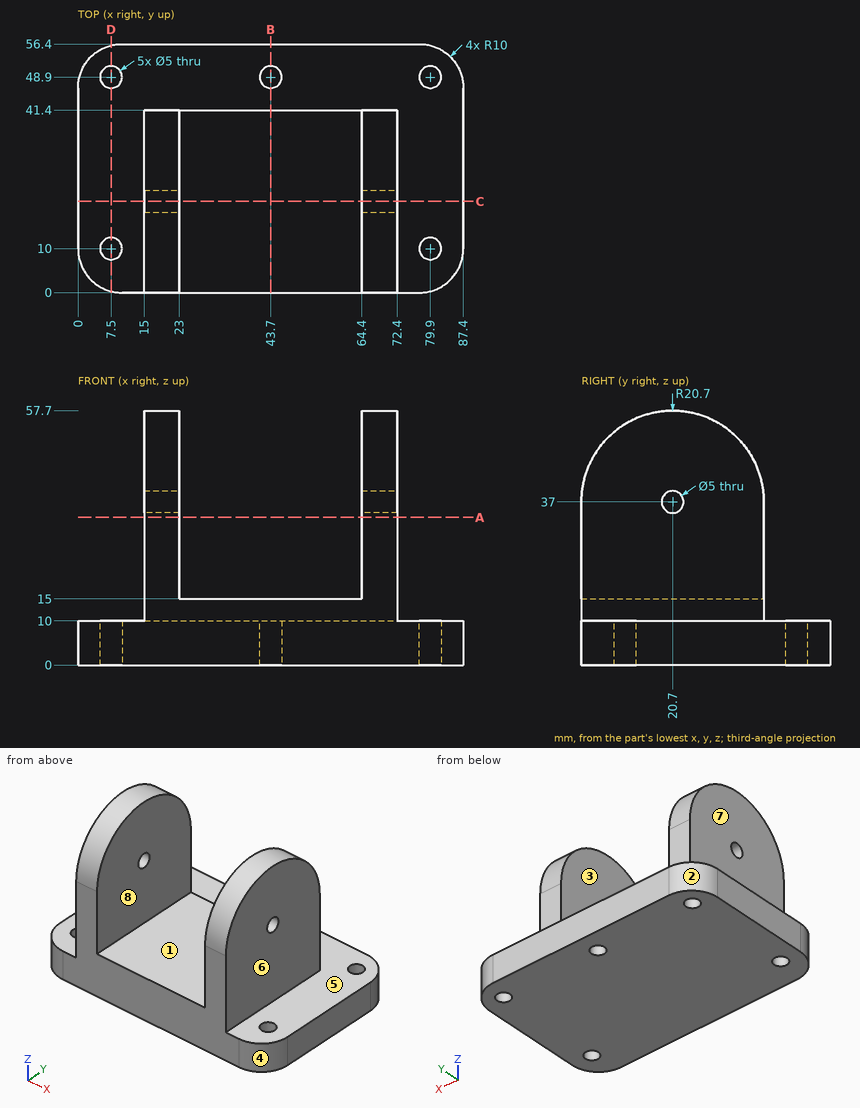
Here's the drawing with two shaded views (mm, measured from the low corner). I have some questions. A direction names the side the tool comes from. Round coordinates to 2 decimals unless told otherwise and drop trailing zeros. Loops run counter-clockwise (first coordinate to the right, second up) from the corner with the lowest first, then second, coordinate; pieces in that order, holes last.
Item 1: Suppose I cut it at B-B, the plane x = 43.7. Write out the boundary of the cut face in (y, z), then the cut area to 3 significant figures.
Item 2: Suppose I cut it at D-D, the plane x = 7.5. Write out the boundary of the cut face in (y, z).
Item 3: Suppose I cut it at C-C, the plane y = 20.7. Write out the boundary of the cut face in (x, z), then the cut area to 3 significant figures.
Item 4: Please list where these lines run through material, in increasing order: L1, parallel to X at y = 22, z = 33; L2, parallel to Y at x = 79.9, z = 2; L3, parallel to Y at x = 7, z = 7.
Item 5: Suppose I cut it at A-A, the plane z = 33.5. Write out the boundary of the cut face in (x, y).
Item 6: If we mould it in two halves opening along X, with no side actions, what happens to the marked faces 1, 2, 3 and 4? For each: +X half, -X half, draft (parallel to the pull), parting line (faces both ways), or undercut.
Item 7: Which directions (+Z, -Z, +X, -X, +Y, -Y) give clear straight access to the entire face, cutting with the end or side of a thin tool? Please do the marked faces 5, 6, 7 and 8.
Item 8: Will these pins go through, and if not, where does the flat tip stop? pin 1 Ø13.5 at (x, z) = (46.5, 19) entering from +Y; pin 2 Ø4.5 at (x, y) = (7.5, 48.9) entering from -Z; pin 3 Ø17 at (x, y) = (23, 17) entering from +Z; pin 4 Ø10 at (x, y) = (64, 38) entering from +Z.
Reported:
1. outline: (0, 0) - (46.4, 0) - (46.4, 10) - (41.4, 10) - (41.4, 15) - (0, 15) - close; (51.4, 0) - (56.4, 0) - (56.4, 10) - (51.4, 10) - close
1. area: 721 mm2
2. outline: (0.32, 0) - (7.5, 0) - (7.5, 10) - (0.32, 10) - close; (12.5, 0) - (46.4, 0) - (46.4, 10) - (12.5, 10) - close; (51.4, 0) - (56.08, 0) - (56.08, 10) - (51.4, 10) - close
3. outline: (0, 0) - (87.4, 0) - (87.4, 10) - (72.4, 10) - (72.4, 34.5) - (64.4, 34.5) - (64.4, 15) - (23, 15) - (23, 34.5) - (15, 34.5) - (15, 10) - (0, 10) - close; (15, 39.5) - (23, 39.5) - (23, 57.7) - (15, 57.7) - close; (64.4, 39.5) - (72.4, 39.5) - (72.4, 57.7) - (64.4, 57.7) - close
3. area: 1,760 mm2
4. L1: x = 15 to 23, 64.4 to 72.4
4. L2: y = 0.32 to 7.5, 12.5 to 46.4, 51.4 to 56.08
4. L3: y = 0.46 to 7.55, 12.45 to 46.45, 51.35 to 55.94
5. outline: (15, 0) - (23, 0) - (23, 41.4) - (15, 41.4) - close; (64.4, 0) - (72.4, 0) - (72.4, 41.4) - (64.4, 41.4) - close
6. face 1: undercut
6. face 2: -X half
6. face 3: undercut
6. face 4: +X half
7. face 5: +Z, +Y
7. face 6: +Z, +X, +Y, -Y
7. face 7: +Z, -X, +Y, -Y
7. face 8: +Z, +Y, -Y
8. pin 1: stops at y = 41.4
8. pin 2: passes through
8. pin 3: stops at z = 57.7
8. pin 4: stops at z = 53.64
